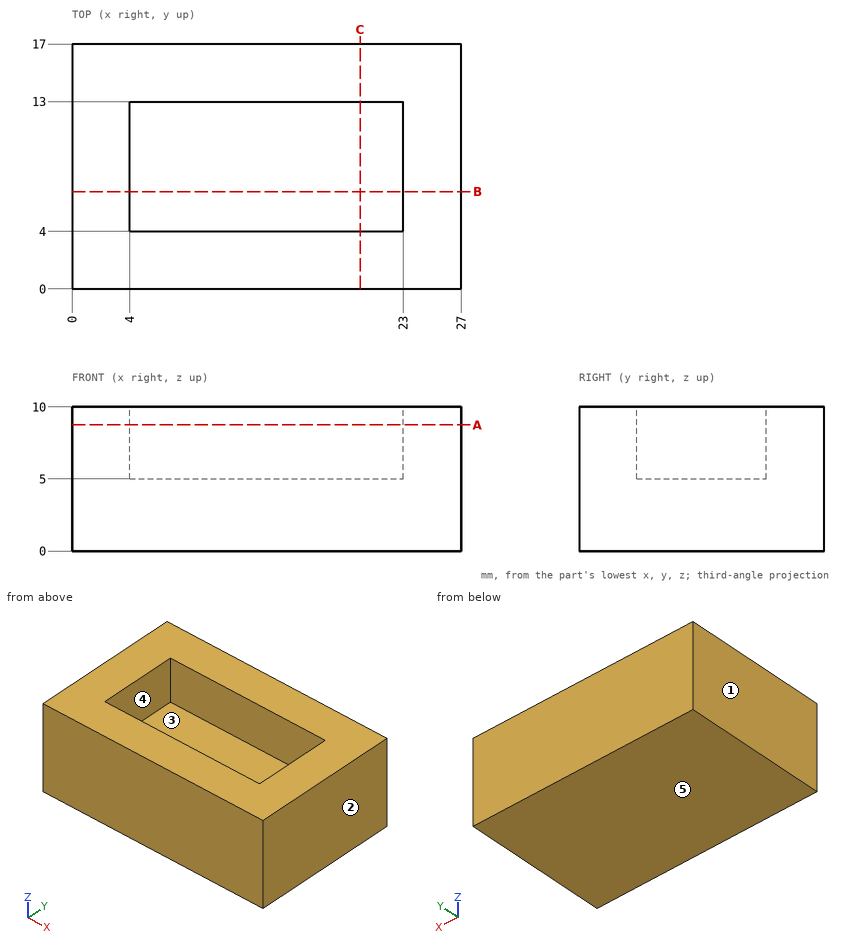
The figure shows three views and two pictorial views of one solid part (mm, origin at its lowest corner). Answer the questions. A direction names the side the tool comes from. Give positions to 0.01 mm unless a question says otherwise; leave off trailing zeros. Order: outer loops, then holes, each group sorted by start corner. A loop starts at its lowest first (then second) coordinate and runs counter-clockwise, first axis right, second up. Notation, with made-up numbers: (70.5, 29.25) -> (119.5, 29.25) arc R18 ccw to (119.5, 40.25) -> close; hole circle Ø2 at (-5, 24.25). An arc over 180 degrees is marked (long way). Answer as CSV lines item,"result". Start each with the question number.
(1) Section B-B, the plane y = 6.75 is taken. Write down the section's boundary in (x, z), plus the area to 3 significant figures.
(2) Consider line 1 along Y through (x, z) = (4.25, 8.25); line 2 along X through (y, z) = (4.75, 6.25); line 3 along Z through (x, y) = (13.25, 7.25). Determine where each line is inside the solid, lowest interval first.
(3) For a pull along X with two mould halves and no side action, classify the marked faces 1, 2 and 3 as released by +X, released by -X, zero draft, split by the parting line, or undercut.
(4) Which of the six approach directions +Z, -Z, +X, -X, +Y, -Y give full straight-line access (tool end or side, diameter ignored) to the marked faces 4 and 5?
(5) Section C-C, the plane x = 20 is taken. Write down the section's boundary in (y, z).
(6) Section A-A, the plane z = 8.75 is taken. Write down the section's boundary in (x, y).
Entries:
1,outline,"(0, 0) -> (27, 0) -> (27, 10) -> (23, 10) -> (23, 5) -> (4, 5) -> (4, 10) -> (0, 10) -> close"
1,area,"175 mm²"
2,line 1,"0 to 4, 13 to 17"
2,line 2,"0 to 4, 23 to 27"
2,line 3,"0 to 5"
3,face 1,"released by -X"
3,face 2,"released by +X"
3,face 3,"undercut"
4,face 4,"+Z"
4,face 5,"-Z, +X, -X, +Y, -Y"
5,outline,"(0, 0) -> (17, 0) -> (17, 10) -> (13, 10) -> (13, 5) -> (4, 5) -> (4, 10) -> (0, 10) -> close"
6,outline,"(0, 0) -> (27, 0) -> (27, 17) -> (0, 17) -> close; hole (4, 4) -> (23, 4) -> (23, 13) -> (4, 13) -> close"
